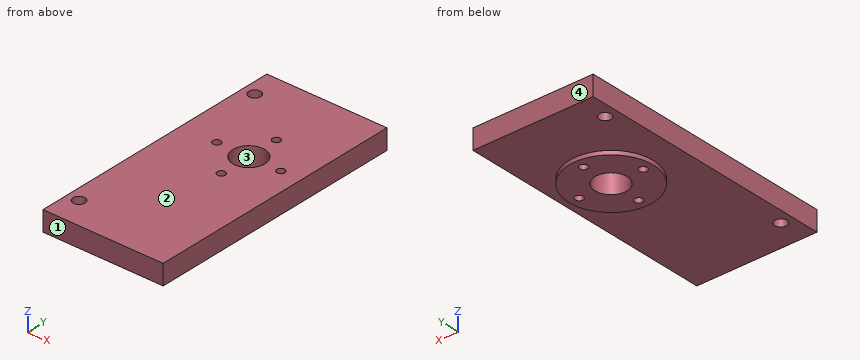
```python
from build123d import *

# Parameters (mm, degrees)
ESQUISSE1_W             = 30
ESQUISSE1_H             = 65
ESQUISSE1_R             = 1.5
ESQUISSE1_R_2           = 1
ESQUISSE1_R_3           = 4
BOSS_EXTRU_1_DEPTH      = 6
ESQUISSE5_W             = 30
ESQUISSE5_H             = 65
ESQUISSE5_R             = 10.5
ENL_V_MAT_EXTRU_4_DEPTH = 1


with BuildPart() as part:
    # Esquisse1 → Boss.-Extru.1 (new body)
    with BuildSketch(Plane.XY):
        with Locations((40.364568032, -83.170745263)):
            Rectangle(ESQUISSE1_W, ESQUISSE1_H)
        with Locations((28.364568032, -57.670745263)):
            Circle(ESQUISSE1_R, mode=Mode.SUBTRACT)
        with Locations((28.364568032, -108.670745263)):
            Circle(ESQUISSE1_R, mode=Mode.SUBTRACT)
        with Locations((34.364568032, -75.670745263)):
            Circle(ESQUISSE1_R_2, mode=Mode.SUBTRACT)
        with Locations((42.364568032, -67.670745263)):
            Circle(ESQUISSE1_R_2, mode=Mode.SUBTRACT)
        with Locations((50.364568032, -75.670745263)):
            Circle(ESQUISSE1_R_2, mode=Mode.SUBTRACT)
        with Locations((42.364568032, -83.670745263)):
            Circle(ESQUISSE1_R_2, mode=Mode.SUBTRACT)
        with Locations((42.364568032, -75.670745263)):
            Circle(ESQUISSE1_R_3, mode=Mode.SUBTRACT)
    extrude(amount=BOSS_EXTRU_1_DEPTH)

    # Esquisse5 → Enlèv. mat.-Extru.4 (cut)
    with BuildSketch(Plane(origin=(0, 0, 0), x_dir=(-1, 0, 0), z_dir=(0, 0, -1))):
        with Locations((-40.364568032, -83.170745263)):
            Rectangle(ESQUISSE5_W, ESQUISSE5_H)
        with Locations((-42.364568032, -75.670745263)):
            Circle(ESQUISSE5_R, mode=Mode.SUBTRACT)
    extrude(amount=-ENL_V_MAT_EXTRU_4_DEPTH, mode=Mode.SUBTRACT)


solid = part.part
```
Input: part model. Units: mm. Frame: model coordinates. Face numbers are marked on the shaded views. Round coordinates to 2 decimals unless told otherwise and drop trailing zeros. Loops run counter-clockwise (first coordinate to the right, second up) from the corner with the lowest first, then second, coordinate; pieces in that order, holes last. Notation, with made-up numbers: (-12, 21) -> (18, 21) arc R12 cw to (18, 35) -> close; hole circle Ø3 at (17, -16). An arc over 180 degrees is marked (long way). Write each question's results on one line, items separated by ' | '.
1. Ray query, line 1 (Y direction, x = 34.5, z = 2.3); line 2 (Y direction, x = 41.5, z = 4.75); line 3 (Z direction, x = 26.75, y = -96.5). Return the intervals inside material, ascending. Write a range as from..to.
Geometry results:
line 1: -115.67..-76.66, -74.68..-50.67 | line 2: -115.67..-84.17, -83.17..-79.58, -71.77..-68.17, -67.17..-50.67 | line 3: 1..6
2. Mould query, pull axis Y, two halves, no side actions, for the marked faces 1, 2, 3 and 4. Classes: +Y half, -Y half, draft (parallel to the pull), parting line (faces both ways), or undercut.
Geometry results:
face 1: -Y half | face 2: draft | face 3: undercut | face 4: +Y half
3. Section C-C (y = -85.5). Return loops of the section in (x, z).
Geometry results:
outline: (25.36, 1) -> (38.67, 1) -> (38.67, 0) -> (46.06, 0) -> (46.06, 1) -> (55.36, 1) -> (55.36, 6) -> (25.36, 6) -> close
4. Section A-A (x = 44). Return loops of the section in (y, z), and give its area (3 significant figures).
Geometry results:
outline: (-115.67, 1) -> (-86.04, 1) -> (-86.04, 0) -> (-79.32, 0) -> (-79.32, 6) -> (-115.67, 6) -> close; (-72.02, 0) -> (-65.3, 0) -> (-65.3, 1) -> (-50.67, 1) -> (-50.67, 6) -> (-72.02, 6) -> close | area: 302 mm2
5. Section D-D (x = 36). Return loops of the section in (y, z), and give its area (3 significant figures).
Geometry results:
outline: (-115.67, 1) -> (-84.02, 1) -> (-84.02, 0) -> (-67.32, 0) -> (-67.32, 1) -> (-50.67, 1) -> (-50.67, 6) -> (-115.67, 6) -> close | area: 342 mm2
6. Section B-B (z = 3.1). Return loops of the section in (x, y).
Geometry results:
outline: (25.36, -115.67) -> (55.36, -115.67) -> (55.36, -50.67) -> (25.36, -50.67) -> close; hole circle Ø3 at (28.36, -108.67); hole circle Ø3 at (28.36, -57.67); hole circle Ø2 at (34.36, -75.67); hole circle Ø8 at (42.36, -75.67); hole circle Ø2 at (42.36, -83.67); hole circle Ø2 at (42.36, -67.67); hole circle Ø2 at (50.36, -75.67)
